Part print with two shaded views. Sizes in mm from the minimum x, y, z corner. A direction names the side the tool comes from. Coordinates: 2 decimals unless noted, no trailing zeros. Order: outer loops, then holes, each group sorted by start corner. A loop starts at its lowest first (then second) coordinate and runs counter-clockwise, first axis right, second up. Notation, with made-up numbers: M 1.25,-10.75 L 5.25,-10.75 A27 ccw 5.25,24.25 Z; hole C 7.25,73.25 d9. An arc over 180 degrees is marked long. Answer in a Markdown table with one row per item. Add a question column.
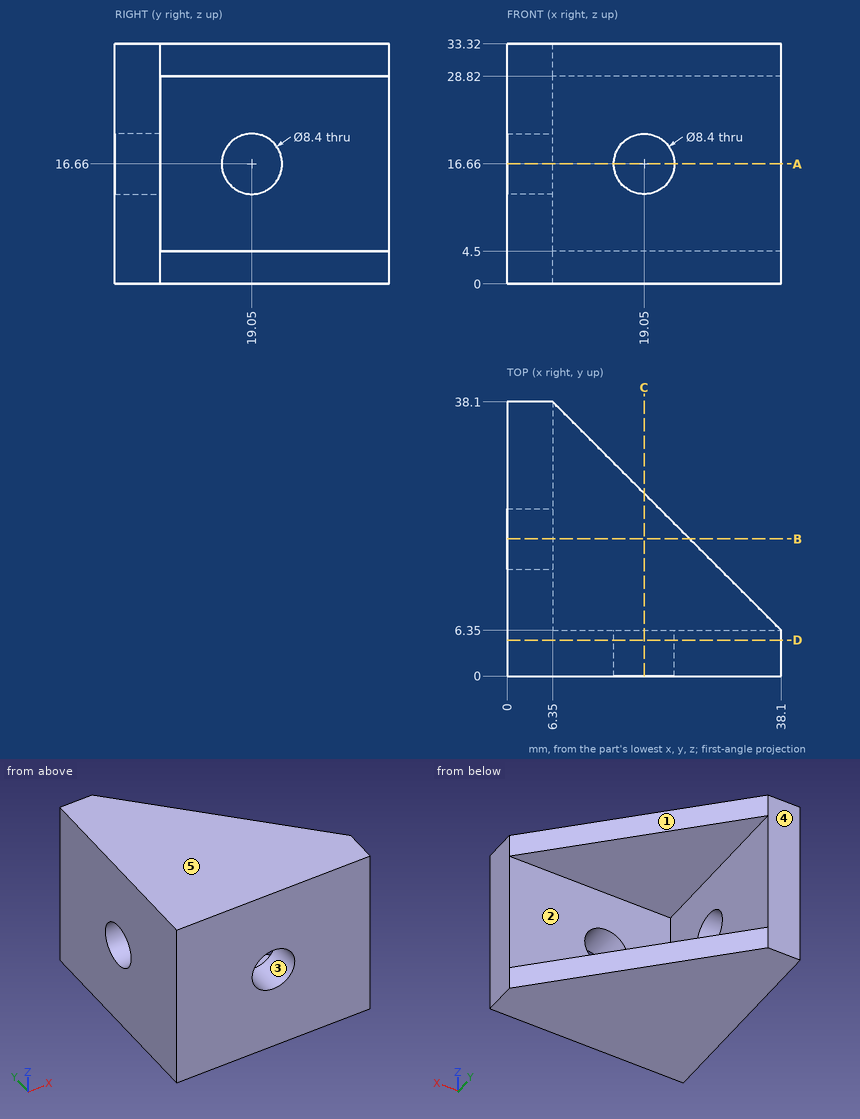
(1) Drop a flat-ended pin along its axis: P1, Ø7.5, axis at y = 22, z = 15.5, coming from the +X side. Give the stop position or say it passes through.
(2) Wall check: line 1 (Z direction, x = 3, y = 19); line 2 (Y direction, x = 30, z = 5). Give the ranges that are in metal, low to high.
(3) 3-axis set-ups, long thin cutter, end or side, ignore diameter. For the marked faces 1 and 2: which of +Z, -Z, +X, -X, +Y, -Y reach the whole face in a straight line?
(4) Slice it at B-B (y = 19.05). List the corners of the cut face in (x, z), and give its area (3 significant figures).
(5) Slice it at A-A (z = 16.66). List the corners of the cut face in (x, y), and give its area (3 significant figures).
(6) Pull direction Z, two halves, no side cores. Call the marked faces 3, 4 and 5: pulls with the +Z half, pulls with the -Z half, needs draft (parallel to the pull), parting line crosses it, or undercut.
(7) Slice it at D-D (y = 5). List the corners of the cut face in (x, z).
Computed:
| question | item | result |
|---|---|---|
| 1 | P1 | stops at x = 6.35 |
| 2 | line 1 | z = 0 to 12.46, 20.86 to 33.32 |
| 2 | line 2 | y = 0 to 6.35 |
| 3 | face 1 | +Z, -Z, +X, +Y |
| 3 | face 2 | +X, +Y |
| 4 | outline | M 0,0 L 25.4,0 L 25.4,4.5 L 6.35,4.5 L 6.35,12.46 L 0,12.46 Z; M 0,20.86 L 6.35,20.86 L 6.35,28.82 L 25.4,28.82 L 25.4,33.32 L 0,33.32 Z |
| 4 | area | 330 mm^2 |
| 5 | outline | M 0,0 L 14.85,0 L 14.85,6.35 L 6.35,6.35 L 6.35,14.85 L 0,14.85 Z; M 0,23.25 L 6.35,23.25 L 6.35,38.1 L 0,38.1 Z; M 23.25,0 L 38.1,0 L 38.1,6.35 L 23.25,6.35 Z |
| 5 | area | 337 mm^2 |
| 6 | face 3 | undercut |
| 6 | face 4 | needs draft |
| 6 | face 5 | pulls with the +Z half |
| 7 | outline | M 0,0 L 38.1,0 L 38.1,33.32 L 0,33.32 Z; hole C 19.05,16.66 d8.4 |
